```python
from build123d import *

# Parameters (mm, degrees)
BOSS_EXTRUDE1_DEPTH = 33
FILLET1_R           = 2


with BuildPart() as part:
    # Sketch1 → Boss-Extrude1 (new body)
    with BuildSketch(Plane(origin=(0, 0, 0), x_dir=(1, 0, 0), z_dir=(0, 1, 0))):
        Polygon((10.5, 1), (10.5, 0), (15, 0), align=None)
        Polygon((15, -5), (15, 0), (0, 0), (0, 18.5), (15, 18.5), (15, 23.5), (-5, 23.5), (-5, -5), align=None)
    extrude(amount=BOSS_EXTRUDE1_DEPTH)

    # Fillet1
    fillet1_edges = [part.edges().sort_by_distance(p)[0] for p in [
        (15, 16.5, 0),
        (-5, 16.5, 5),
        (-5, 16.5, -23.5),
        (15, 16.5, -23.5),
        (15, 16.5, -18.5),
        (0, 16.5, -18.5),
        (0, 16.5, 0),
    ]]
    fillet(fillet1_edges, radius=FILLET1_R)


solid = part.part
```
Could you check a few things on this model? Use its own coordinates, in mm. A direction names the side the tool comes from. Coordinates: 2 decimals unless noted, no trailing zeros. Order: outer loops, then holes, each group sorted by start corner. A loop starts at its lowest first (then second) coordinate and runs counter-clockwise, first axis right, second up. Notation, with made-up numbers: M 5.25,35 L 10.25,35 A26 cw 10.25,71 Z; hole C 54,75.25 d8. An arc over 180 degrees is marked long. Use one line per item in the form item = value. Start each with the question number.
1. Suppose I cut it at C-C on x = 1. Write out the boundary of the cut face in (y, z), then the cut area to 3 significant figures.
2. For pin 1 (10 mm diameter, centred on x = 7, z = -7.5, fed in from -Y); pin 2 (1 mm diameter, centred on y = 26, z = -13, fed in from +X), each with a flat end and sliding along its axis, tell me the tip position at first contact or that it passes through.
3. Suppose I cut it at A-A on x = 9.75. Write out the boundary of the cut face in (y, z), then the cut area to 3 significant figures.
4. Suppose I cut it at D-D on z = -4. Write out the boundary of the cut face in (x, y).
5. We'd pull the mould along X, two halves only. Please class faces 4 (the cylindrical face through (14.43, 16.73, -22.9)), 5 (the flat face through (10.5, 16.3, -0.5)), 6 (the flat face through (-5, 16, -9)): +X half, -X half, draft (parallel to the pull), parting line (faces both ways), or undercut.
6. Suppose I cut it at B-B on y = 30. Write out the boundary of the cut face in (x, z).
7. On a 3-axis mill with a long thin cutter (end or side, diameter ignored), from which of +Z, -Z, +X, -X, +Y, -Y can I reach the whole of each face in a straight line? I mean faces 1 (the cylindrical face through (14.572, 16.731, 0.368)), 2 (the flat face through (6, 16, 0)), 3 (the flat face through (-2, 33, -9)). Say none if no direction works.
8. Please list where these lines run through material, in increasing order: line 1 (Z direction, x = 8.5, y = 26); line 2 (X direction, y = 5, z = -8.25); line 3 (Z direction, x = 10.75, y = 30).
Geometry says:
q1.outline = M 0,-23.5 L 33,-23.5 L 33,-18.23 L 0,-18.23 Z; M 0,-0.27 L 33,-0.27 L 33,5 L 0,5 Z
q1.area = 348 mm^2
q2.pin_1 = through
q2.pin_2 = 0
q3.outline = M 0,-23.5 L 33,-23.5 L 33,-18.5 L 0,-18.5 Z; M 0,0 L 33,0 L 33,5 L 0,5 Z
q3.area = 330 mm^2
q4.outline = M -5,0 L 0,0 L 0,33 L -5,33 Z
q5.face_4 = +X half
q5.face_5 = undercut
q5.face_6 = -X half
q6.outline = M -5,-21.5 A2 ccw -3,-23.5 L 13,-23.5 A2 ccw 15,-21.5 L 15,-20.5 A2 ccw 13,-18.5 L 2,-18.5 A2 cw 0,-16.5 L 0,-2 A2 cw 2,0 L 10.5,0 L 10.5,-1 L 13.43,-0.35 A2 ccw 15,1.6 L 15,5 L -3,5 A2 ccw -5,3 Z
q7.face_1 = +X, +Y, -Y
q7.face_2 = +Y, -Y
q7.face_3 = +Z, -Z, +X, -X, +Y
q8.line_1 = -23.5 to -18.5, 0 to 5
q8.line_2 = -5 to 0
q8.line_3 = -23.5 to -18.5, -0.94 to 5
